CAD build for the part. Positions are in the model's coordinates, mm. Face numbers are marked on the shaded views. A direction names the side the tool comes from. Coordinates: 2 decimals unless noted, no trailing zeros. Order: outer loops, then holes, each group sorted by start corner. A loop starts at its lowest first (then second) coordinate and runs counter-clockwise, first axis right, second up. Notation, with made-up numbers: M 59,-35.5 L 105,-35.5 A11 cw 105,-28.5 Z; hole C 34.5,-31.75 d8. An arc over 180 degrees is marked long. Write item = value, one per line.
from build123d import *

# Parameters (mm, degrees)
F0_R      = 12.400699
F1_DEPTH  = 34.005828
F2_R      = 12.950879
F3_DEPTH  = 32.92565
F5_W      = 24.064958
F5_H      = 32.778248
F6_DEPTH  = 60.947001
F4_W      = 26.554584
F4_H      = 23.65014
F8_DEPTH  = 25.4
F7_R      = 6.344063
F9_DEPTH  = 14.975553
F10_R     = 7.426206
F11_DEPTH = 16.588198
F12_R     = 16.389124
F13_DEPTH = 61.027274


with BuildPart() as f1:
    # F0 (on Right) → F1 (new body)
    with BuildSketch(Plane.YZ):
        Circle(F0_R)
    extrude(amount=F1_DEPTH)

    # F2 (on Right) → F3 (join)
    with BuildSketch(Plane.YZ):
        Circle(F2_R)
    extrude(amount=-F3_DEPTH)

    # F5 (on Top) → F6 (join)
    with BuildSketch(Plane.XY):
        Rectangle(F5_W, F5_H)
    extrude(amount=-F6_DEPTH)

    # F4 (on Top) → F8 (join)
    with BuildSketch(Plane.XY):
        Rectangle(F4_W, F4_H)
    extrude(amount=F8_DEPTH)

    # F7 (on face) → F9 (join)
    with BuildSketch(Plane.YZ.offset(34.005828)):
        Circle(F7_R)
    extrude(amount=F9_DEPTH)

    # F10 (on face) → F11 (join)
    with BuildSketch(Plane(origin=(-32.92565, 0, 0), x_dir=(0, -1, 0), z_dir=(-1, 0, 0))):
        Circle(F10_R)
    extrude(amount=F11_DEPTH)

    # F12 (on face) → F13 (join)
    with BuildSketch(Plane(origin=(0, 0, -60.947001), x_dir=(1, 0, 0), z_dir=(0, 0, -1))):
        with BuildLine():
            Line((12.032479, -11.127571), (12.032479, 11.127571))
            ThreePointArc((12.032479, 11.127571), (6.566287, 15.016233), (0, 16.389124))
            ThreePointArc((0, 16.389124), (-6.566287, 15.016233), (-12.032479, 11.127571))
            Line((-12.032479, 11.127571), (-12.032479, -11.127571))
            ThreePointArc((-12.032479, -11.127571), (-6.566287, -15.016233), (0, -16.389124))
            ThreePointArc((0, -16.389124), (6.566287, -15.016233), (12.032479, -11.127571))
        make_face()
        Circle(F12_R)
    extrude(amount=F13_DEPTH)


solid = f1.part
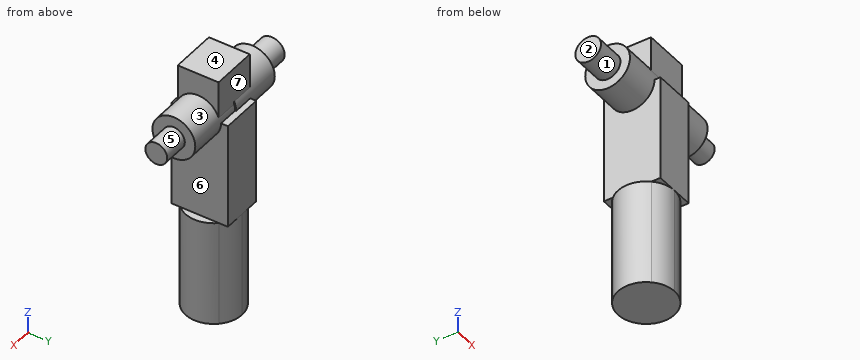
(1) Pull direction Z, two halves, no side cores. Call the marked faces 4, 5, 6 and 7: +Z half, -Z half, draft (parallel to the pull), parting line (faces both ways), or undercut.
Evaluation:
face_4 = +Z half
face_5 = parting line
face_6 = undercut
face_7 = draft
(2) Tool access for the marked faces 1, 2 and 3: list every direction of +Z, -Z, +X, -X, +Y, -Y with a clear straight run to the whole face (end or side of a thin tool).
Evaluation:
face_1 = -X
face_2 = +Z, -Z, -X, +Y, -Y
face_3 = +X
(3) Slice it at D-D, the plane z = -58.5. Write the cut outline in (x, y).
Evaluation:
outline = M -12.03,-16.39 L 12.03,-16.39 L 12.03,16.39 L -12.03,16.39 Z
(4) Slice it at A-A, the plane y = 0. Write the cut outline in (x, z).
Evaluation:
outline = M -49.51,-7.43 L -32.93,-7.43 L -32.93,-12.95 L -12.03,-12.95 L -12.03,-60.95 L -16.39,-60.95 L -16.39,-121.97 L 16.39,-121.97 L 16.39,-60.95 L 12.03,-60.95 L 12.03,-12.4 L 34.01,-12.4 L 34.01,-6.34 L 48.98,-6.34 L 48.98,6.34 L 34.01,6.34 L 34.01,12.4 L 13.28,12.4 L 13.28,25.4 L -13.28,25.4 L -13.28,12.95 L -32.93,12.95 L -32.93,7.43 L -49.51,7.43 Z
(5) Pin check, flat tips, straight feed: pin 1 Ø2 at (x, y) = (31, -9.5) entering from +Z; pin 2 Ø8 at (y, z) = (4, -96) entering from +X; pin 3 Ø6 at (y, z) = (-7, -101.5) entering from -X. Stop position of each tip, or through.
Evaluation:
pin_1 = 9.03
pin_2 = 16.39
pin_3 = -15.89
(6) Slice it at B-B, the plane z = -107. Write the cut outline in (x, y).
Evaluation:
outline = M -12.03,-11.13 A16.39 ccw 0,-16.39 A16.39 ccw 12.03,-11.13 A16.39 ccw 12.03,11.13 A16.39 ccw 0,16.39 A16.39 ccw -12.03,11.13 A16.39 ccw Z
(7) Slice it at C-C, the plane x = 6.5. Write the cut outline in (y, z).
Evaluation:
outline = M -16.39,-60.95 L -15.05,-60.95 L -15.05,-121.97 L 15.05,-121.97 L 15.05,-60.95 L 16.39,-60.95 L 16.39,0 L 12.4,0 A12.4 ccw 11.83,3.73 L 11.83,25.4 L -11.83,25.4 L -11.83,3.73 A12.4 ccw -12.4,0 L -16.39,0 Z
(8) Wall check: line 1 (X direction, y = 1, z = -96); line 2 (Z direction, x = 33, y = 5.5); line 3 (X direction, y = 10, z = -114). Give the ranges that are in metal, low to high. Write a range as from..to.
Evaluation:
line_1 = -16.36..16.36
line_2 = -11.11..11.11
line_3 = -12.98..12.98
